For this review, use the dimensioned drawing (mm, ordinates from the lowest corner) and the shaded views. A direction names the side the tool comes from. Give positions to 0.01 mm unless a question says otherwise; leave off trailing zeros. Write each loop counter-clockwise with the first axis right and the second up, starting at its lowest first coordinate (ties: lowest second). Pieces come first, ordered by that corner, then holes. Notation, with made-up numbers: (1, 10.5) - (15, 10.5) arc R13 cw to (15, 14.5) - close; hole circle Ø4 at (73.25, 14.5). An arc over 180 degrees is marked (long way). Use a Markdown table: item, result. Add a question column.
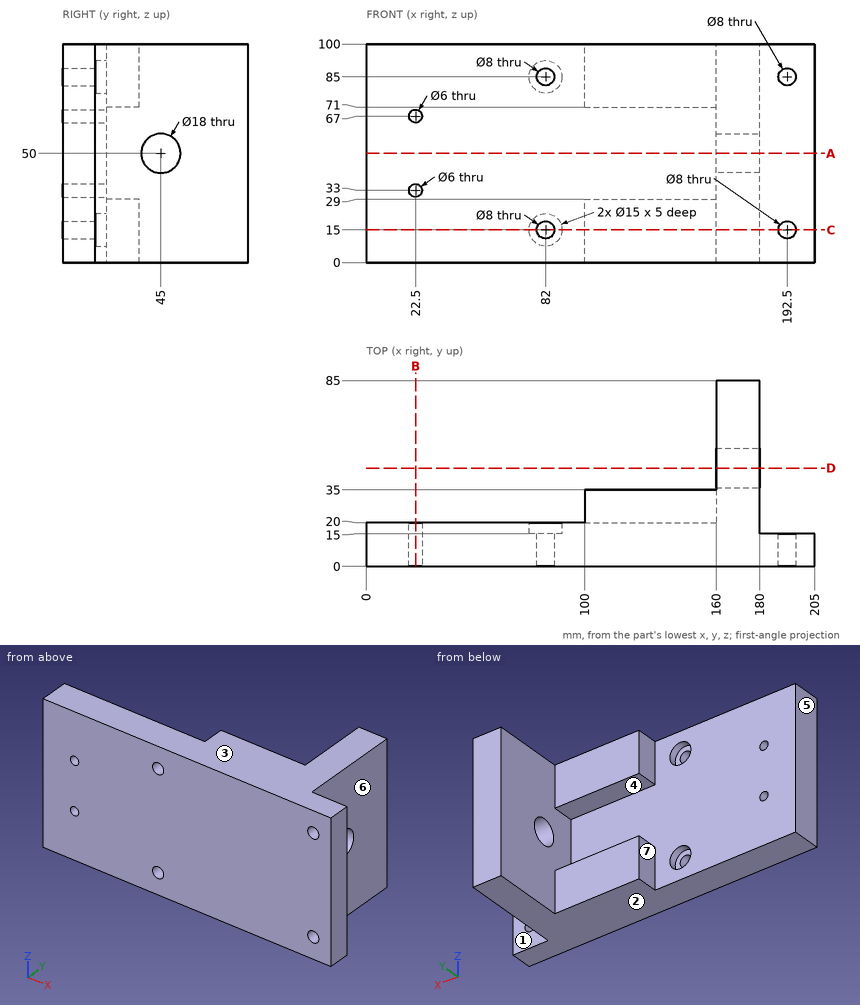
(1) Tool access review of the marked faces 5, 6 and 7: name each direction out of +Z, -Z, +X, -X, +Y, -Y from which nothing blocks a thin tool from reaching the whole face with its end or side.
(2) Insertion check: pin 1 (10.5 mm diameter, centred on x = 192.5, z = 15, fed in from -Y); pin 2 (12 mm diameter, centred on y = 28, z = 7.5, fed in from -X); pin 3 (6.5 mm diameter, centred on x = 82, z = 85, fed in from +Y); pin 4 (4 mm diameter, centred on x = 117.5, z = 55.5, fed in from +Y). Each pin has a flat end and moves straight along its axis. Give the tip position at first contact, or say it passes through.
(3) Mouldability with a two-part tool opening along Z and no side actions: class the marked faces 1, 2, 3 and 4 as +Z half, -Z half, draft (parallel to the pull), parting line (faces both ways), or undercut.
(4) Add section B-B (x = 22.5). State the section outline as (y, z) points.
(5) Add section C-C (z = 15). State the section outline as (x, y) points, and give its area (3 significant figures).
(6) For line 1 along Z through (x, y) = (192.5, 7); line 2 along Z through (x, y) = (82, 18.5); line 3 along X through (y, z) = (9, 33), list the stretches that pass through material, from the lowest coordinate up.
(7) Add section D-D (y = 45). State the section outline as (x, z) points.
(8) Add section A-A (z = 50). State the section outline as (x, y) points, and give its area (4 significant figures).
Answers follow:
| question | item | result |
|---|---|---|
| 1 | face 5 | +Z, -Z, -X, +Y, -Y |
| 1 | face 6 | +Z, -Z, +X, +Y |
| 1 | face 7 | +Z, -Z, -X, +Y |
| 2 | pin 1 | y = 0 |
| 2 | pin 2 | x = 100 |
| 2 | pin 3 | through |
| 2 | pin 4 | y = 20 |
| 3 | face 1 | draft |
| 3 | face 2 | -Z half |
| 3 | face 3 | +Z half |
| 3 | face 4 | undercut |
| 4 | outline | (0, 0) - (20, 0) - (20, 30) - (0, 30) - close; (0, 36) - (20, 36) - (20, 64) - (0, 64) - close; (0, 70) - (20, 70) - (20, 100) - (0, 100) - close |
| 5 | outline | (0, 0) - (78, 0) - (78, 15) - (74.5, 15) - (74.5, 20) - (0, 20) - close; (86, 0) - (188.5, 0) - (188.5, 15) - (180, 15) - (180, 85) - (160, 85) - (160, 35) - (100, 35) - (100, 20) - (89.5, 20) - (89.5, 15) - (86, 15) - close; (196.5, 0) - (205, 0) - (205, 15) - (196.5, 15) - close |
| 5 | area | 5,860 mm^2 |
| 6 | line 1 | 0 to 11, 19 to 81, 89 to 100 |
| 6 | line 2 | 0 to 7.5, 22.5 to 77.5, 92.5 to 100 |
| 6 | line 3 | 0 to 19.5, 25.5 to 205 |
| 7 | outline | (160, 0) - (180, 0) - (180, 41) - (160, 41) - close; (160, 59) - (180, 59) - (180, 100) - (160, 100) - close |
| 8 | outline | (0, 0) - (205, 0) - (205, 15) - (180, 15) - (180, 36) - (160, 36) - (160, 20) - (0, 20) - close; (160, 54) - (180, 54) - (180, 85) - (160, 85) - close |
| 8 | area | 4,915 mm^2 |
